Could you check a few things on this model? Use its own coordinates, in mm. Face numbers are marked on the shaded views. A direction names the side the tool comes from. Round coordinates to 2 decimals unless told otherwise and drop trailing zeros. Loops run counter-clockwise (first coordinate to the right, second up) from the corner with the lowest first, then second, coordinate; pieces in that order, holes last. Notation, with made-up numbers: (6, 63) -> (18, 63) arc R15 ccw to (18, 76) -> close; hole circle Ø7 at (12.25, -18.5). An arc over 180 degrees is marked (long way). Write each question's results on one line, items separated by ' | '. Start each with the question number.
1) Which directions (+Z, -Z, +X, -X, +Y, -Y) give clear straight access to the entire face, cutting with the end or side of a thin tool? Please do the marked faces 1, 2 and 3.
2) Imagine slicing it at A-A, the plane x = 0. Give the number of separate pieces and of enclosed holes in the cut face, plus the area to 3 significant figures.
3) Imagine slicing it at C-C, the plane y = -4.6. List the corners of the cut face in (x, z) for me.
4) If I drill on probe 1 along X at (y, z) = (23.05, 41.5); probe 2 along Z at (x, y) = (-11.4, 25.6); probe 3 along X at (y, z) = (25, 44), over which ranges is the centre line in solid material (lowest first)?
5) Imagine slicing it at B-B, the plane z = 14.5. List the corners of the cut face in (x, y) for me.
6) Imagine slicing it at D-D, the plane x = -11.4. List the corners of the cut face in (y, z) for me, plus the area to 3 significant figures.
7) For P1, Ø6, axis at x = -11, z = 17.5, coming from the -Y side; P2, Ø5, axis at y = -4.6, z = 31, coming from the +X side; P3, Ø6, axis at x = 9, y = -5.5, coming from the -Z side; P4, Ø3.5, axis at x = -11.4, z = 41.5, coming from the +Y side, each with a flat end and sliding along its axis, tell me the tip position at first contact or that it passes through.
Autodesk Inventor part; units mm, degrees
ref_plane "YZ Plane" through (0, 0, 0) normal (1, 0, 0) x (0, 1, 0)
ref_plane "XZ Plane" through (0, 0, 0) normal (0, 1, 0) x (-1, 0, 0)
ref_plane "XY Plane" through (0, 0, 0) normal (0, 0, 1) x (1, 0, 0)
sketch "Skizze1" plane through (0, 0, 0) normal (0, 0, 1) x (1, 0, 0)
  line L0 (-19, 27.1) -> (19, 27.1)
  line L1 (19, 27.1) -> (19, -27.1)
  line L2 (19, -27.1) -> (-19, -27.1)
  line L3 (-19, -27.1) -> (-19, 27.1)
  line L4 (0, 37.94) -> (0, -37.94)
  line L5 (-26.6, 0) -> (26.6, 0)
  point P0 (0, 0)
  dimension "d0" = 38
  dimension "d1" = 54.2
  dimension "d46" = 19
  dimension "d47" = 27.1
extrude "Extrusion1" add sketch "Skizze1" along normal blind 63
sketch "Skizze2" plane through (0, 0, 63) normal (0, 0, 1) x (1, 0, 0)
  line L0 (-19, -27.1) -> (19, -27.1)
  line L1 (-19, -27.1) -> (19, -27.1)
  line L2 (19, -27.1) -> (19, 21.1)
  line L3 (19, 21.1) -> (-19, 21.1)
  line L4 (-19, 21.1) -> (-19, -27.1)
  line L5 (-19, 27.1) -> (-19, -27.1)
  line L6 (19, 27.1) -> (-19, 27.1)
  point P0 (0, 0)
  dimension "d4" = 38
  dimension "d6" = 6
extrude "Extrusion2" cut sketch "Skizze2" against normal through all
sketch "Skizze6" plane through (-19, 27.1, 0) normal (0, 1, 0) x (1, 0, 0)
  line L0 (38, -63) -> (0, -63)
  line L1 (38, 0) -> (0, 0)
  line L2 (19, 12.6) -> (19, -75.6)
  point P0 (19, 0)
  point P1 (19, -44)
  point P2 (19, -19)
  dimension "d48" = 25
  dimension "d49" = 63
  dimension "d50" = 19
hole "Bohrung4" at (0, 27.1, 44) at (0, 27.1, 19) direction (0, -1, 0) diameter 5 depth 2.5
sketch "Skizze13" plane through (-19, 21.1, 63) normal (0, -1, 0) x (1, 0, 0)
  line L0 (38, 0) -> (38, -63)
  line L1 (0, -63) -> (0, 0)
  line L2 (38, -63) -> (0, -63)
  line L3 (0, 0) -> (38, 0)
  point P0 (19, -63)
  point P1 (7.6, -21.5)
  point P2 (27.6, -21.5)
  point P3 (27.6, -41.5)
  point P4 (7.6, -41.5)
  dimension "d102" = 20
  dimension "d103" = 20
  dimension "d104" = 38
  dimension "d105" = 7.6
  dimension "d106" = 63
  dimension "d107" = 21.5
hole "Bohrung6" at (-11.4, 21.1, 41.5) at (8.6, 21.1, 41.5) at (8.6, 21.1, 21.5) at (-11.4, 21.1, 21.5) direction (0, 1, 0) diameter 4.5 end through all counterbore diameter 8 counterbore depth 4
sketch "Skizze14" plane through (0, 0, 63) normal (0, 0, 1) x (1, 0, 0)
  line L0 (19, 27.1) -> (-19, 27.1)
  line L1 (-19, 27.1) -> (19, 27.1)
  line L2 (19, 27.1) -> (19, -27.1)
  line L3 (19, -27.1) -> (-19, -27.1)
  line L4 (-19, -27.1) -> (-19, 27.1)
  line L5 (19, 21.1) -> (19, 27.1)
  point P0 (0, 0)
  dimension "d115" = 54.2
extrude "Extrusion8" add sketch "Skizze14" along normal blind 5
sketch "Skizze15" plane through (0, 0, 68) normal (0, 0, -1) x (-1, 0, 0)
  line L0 (-19, 21.1) -> (19, 21.1)
  line L1 (3.3, 13.4) -> (-3.3, 13.4)
  line L2 (-3.3, 13.4) -> (-3.3, 6.8)
  line L3 (-3.3, 6.8) -> (3.3, 6.8)
  line L4 (3.3, 6.8) -> (3.3, 13.4)
  line L5 (3.3, 13.4) -> (-3.3, 6.8) construction
  line L6 (-3.3, 13.4) -> (3.3, 6.8) construction
  arc A0 (3.3, 6.8) -> (3.3, 13.4) centre (3.3, 10.1) ccw
  arc A1 (-3.3, 13.4) -> (-3.3, 6.8) centre (-3.3, 10.1) ccw
  line L7 (3.3, -22.2) -> (-3.3, -22.2)
  line L8 (-3.3, -22.2) -> (-3.3, -15.6)
  line L9 (-3.3, -15.6) -> (3.3, -15.6)
  line L10 (3.3, -15.6) -> (3.3, -22.2)
  line L11 (3.3, -22.2) -> (-3.3, -15.6) construction
  line L12 (-3.3, -22.2) -> (3.3, -15.6) construction
  arc A2 (3.3, -22.2) -> (3.3, -15.6) centre (3.3, -18.9) ccw
  arc A3 (-3.3, -15.6) -> (-3.3, -22.2) centre (-3.3, -18.9) ccw
  point P0 (0, 0)
  point P1 (0, 10.1)
  point P2 (0, -18.9)
  dimension "d118" = 11
  dimension "d119" = 29
  dimension "d149" = 6.6
  dimension "d150" = 6.6
  dimension "d151" = 6.6
  dimension "d152" = 6.6
  dimension "d153" = 3.3
sketch "Sketch17" plane through (19, 21.1, 0) normal (1, 0, 0) x (0, 0, -1)
  line L0 (-68, -48.2) -> (0, -48.2)
  line L1 (0, -48.2) -> (0, -1)
  line L2 (0, -1) -> (-68, -1)
  line L3 (-68, -1) -> (-68, -48.2)
  line L4 (-63, 0) -> (0, 0)
  dimension "d137" = 1
extrude "Extrusion9" [suppressed]
sketch "Sketch21" plane through (-19, 21.1, 0) normal (-1, 0, 0) x (0, 0, 1)
  line L0 (63, -48.2) -> (68, -48.2)
  line L1 (68, -48.2) -> (0, -48.2)
  line L2 (0, -48.2) -> (0, -3.2)
  line L3 (0, -3.2) -> (68, -3.2)
  line L4 (68, -3.2) -> (68, -48.2)
  point P0 (0, -21.1)
  dimension "d170" = 45
extrude "Extrusion12" add sketch "Sketch21" along normal blind 6
fillet "Fillet2" radius 6 2 edges at (0, 27.1, 68) (-25, -4.6, 68)
extrude "Extrusion10" cut sketch "Skizze15" along normal blind 6
sketch "Sketch19" plane through (0, 0, 63) normal (0, 0, -1) x (-1, 0, 0)
  arc A0 (3.3, -22.2) -> (3.3, -15.6) centre (3.3, -18.9) ccw
  line L0 (3.3, -22.2) -> (-3.3, -22.2)
  arc A1 (-3.3, -15.6) -> (-3.3, -22.2) centre (-3.3, -18.9) ccw
  line L1 (-3.3, -15.6) -> (3.3, -15.6)
  line L2 (-3.3, 13.4) -> (3.3, 13.4)
  arc A2 (3.3, 6.8) -> (3.3, 13.4) centre (3.3, 10.1) ccw
  line L3 (3.3, 6.8) -> (-3.3, 6.8)
  arc A3 (-3.3, 13.4) -> (-3.3, 6.8) centre (-3.3, 10.1) ccw
  line L4 (19, 21.1) -> (-19, 21.1)
  line L5 (-19, -27.1) -> (-19, 21.1)
  line L6 (19, -27.1) -> (-19, -27.1)
  line L7 (19, 21.1) -> (19, 17.9)
  line L8 (-9.0001, 14.625) -> (8.9999, 14.625)
  line L9 (8.9999, 14.625) -> (8.9999, 5.625)
  line L10 (8.9999, 5.625) -> (-9.0001, 5.625)
  line L11 (-9.0001, 5.625) -> (-9.0001, 14.625)
  line L12 (-9.0001, 14.625) -> (8.9999, 5.625) construction
  line L13 (8.9999, 14.625) -> (-9.0001, 5.625) construction
  circle A4 centre (4.4999, 10.125) radius 4.5
  circle A5 centre (-4.5001, 10.125) radius 4.5
  line L14 (-9.0001, -14.4) -> (8.9999, -14.4)
  line L15 (8.9999, -14.4) -> (8.9999, -23.4)
  line L16 (8.9999, -23.4) -> (-9.0001, -23.4)
  line L17 (-9.0001, -23.4) -> (-9.0001, -14.4)
  line L18 (-9.0001, -14.4) -> (8.9999, -23.4) construction
  line L19 (8.9999, -14.4) -> (-9.0001, -23.4) construction
  circle A6 centre (4.4999, -18.9) radius 4.5
  circle A7 centre (-4.5001, -18.9) radius 4.5
  arc A8 (-3.3, -15.6) -> (-3.3, -22.2) centre (-3.3, -18.9) ccw
  line L20 (19, 17.9) -> (19, -27.1)
  point P0 (0, 0)
  point P1 (-0.0001, 10.125)
  point P2 (-0.1415, -24.1318)
  point P3 (-0.0001, -18.9)
  point P4 (-0.1415, -22.2)
  point P5 (-4.5001, -23.4)
  point P6 (4.4999, -23.4)
  point P7 (4.4999, -14.4)
  point P8 (-4.5001, -14.4)
  point P9 (-4.5001, 5.625)
  point P10 (4.4999, 5.625)
  point P11 (4.4999, 14.625)
  point P12 (-4.5001, 14.625)
  dimension "d156" = 18
  dimension "d157" = 9
  dimension "d158" = 9
  dimension "d160" = 18
  dimension "d161" = 9
  dimension "d162" = 9
  dimension "d165" = 9
  dimension "d166" = 1.2001
  dimension "d167" = 1.2001
extrude "Extrusion11" cut sketch "Sketch19" against normal blind 2 contours A0 L1 A6 L0 | A6 L16 A7 L0 | L1 A7 L14 A6 | A7 L1 A1 L0 | A3 L3 A5 L2 | A5 L8 A4 L2 | A4 L3 A2 L2 | L3 A4 L10 A5 picked at (8.1543, -18.4336) picked at (-8.1544, -18.4336) picked at (-8.1544, 10.583) picked at (8.1543, 10.583)
sketch "Sketch22" plane through (-25, 21.1, 0) normal (-1, 0, 0) x (0, 0, 1)
  line L0 (0, -48.2) -> (62, -48.2)
  point P0 (0, -21.1)
  point P1 (31, -25.7)
  point P2 (31, -48.2)
  dimension "d173" = 0
  dimension "d174" = 22.5
sketch "Sketch18" plane through (25, 21.1, 0) normal (1, 0, 0) x (0, 0, -1)
  line L0 (-62, -48.2) -> (0, -48.2)
  line L1 (0, -1) -> (-62, -1)
  point P0 (0, -21.1)
  point P1 (-34.0313, -24.6)
  dimension "d139" = 23.6
  dimension "d140" = 47.2
hole "Hole9" [suppressed]
hole "Hole10" at (-25, -4.6, 31) direction (1, 0, 0) diameter 4.134 end through all
equation "\"d46\" = 0.5 * d0"
equation "\"d47\" = 0.5 * d1"
equation "\"d167\" = d166"
properties part number "TS_Adapter_Greifer_int"
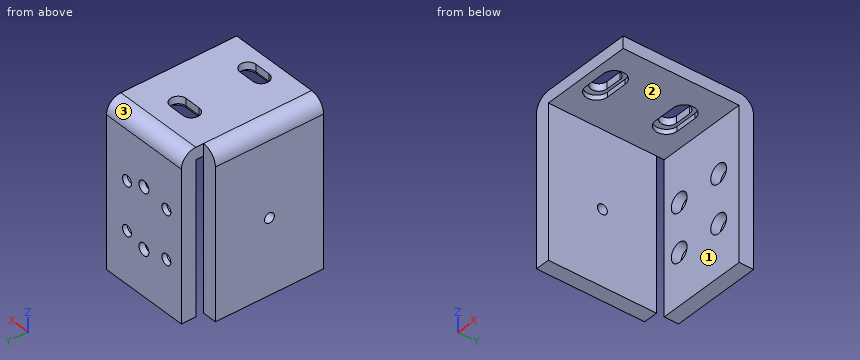
Checked values:
1) face 1: -Z, +X, -X, -Y | face 2: -Z, +X, -Y | face 3: +Z, +X, -X, +Y
2) separate pieces: 3 | enclosed holes: 0 | area: 541 mm^2
3) outline: (-25, 0) -> (-19, 0) -> (-19, 28.93) -> (-25, 28.93) -> close; (-25, 33.07) -> (-19, 33.07) -> (-19, 63) -> (19, 63) -> (19, 68) -> (-19, 68) arc R6 ccw to (-25, 62) -> close
4) probe 1: -19 to -15.4, -7.4 to 4.6, 12.6 to 19 | probe 2: 0 to 19.25, 23.75 to 39.25, 43.75 to 65.97 | probe 3: -19 to -14.52, -8.28 to -2.5, 2.5 to 5.48, 11.72 to 19
5) outline: (-25, -27.1) -> (-19, -27.1) -> (-19, 17.9) -> (-25, 17.9) -> close; (-19, 21.1) -> (19, 21.1) -> (19, 27.1) -> (-19, 27.1) -> close
6) outline: (-27.1, 63) -> (21.1, 63) -> (21.1, 45.5) -> (25.1, 45.5) -> (25.1, 43.75) -> (27.1, 43.75) -> (27.1, 62) arc R6 ccw to (21.1, 68) -> (-27.1, 68) -> close; (21.1, 0) -> (27.1, 0) -> (27.1, 19.25) -> (25.1, 19.25) -> (25.1, 17.5) -> (21.1, 17.5) -> close; (21.1, 25.5) -> (25.1, 25.5) -> (25.1, 23.75) -> (27.1, 23.75) -> (27.1, 39.25) -> (25.1, 39.25) -> (25.1, 37.5) -> (21.1, 37.5) -> close | area: 559 mm^2
7) P1: y = 21.1 | P2: x = -19 | P3: z = 63 | P4: through
